Design review of the part shown in the three views and the two pictorial views. Dimensions are in mm from the part's minimum x, y and z. A direction names the side the tool comes from. Round coordinates to 2 decimals unless told otherwise and drop trailing zeros. Order: outer loops, then holes, each group sorted by start corner. A loop starts at its lowest first (then second) coordinate and runs counter-clockwise, first axis right, second up.
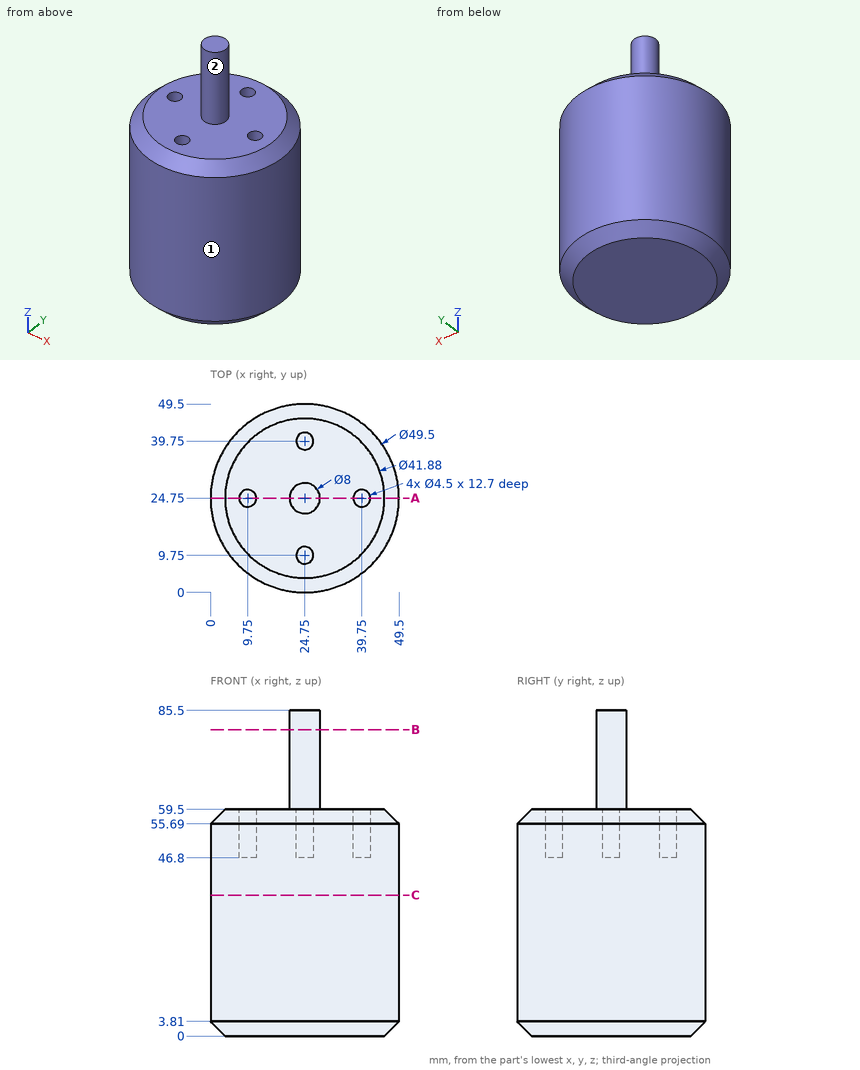
(1) Insertion check: pin 1 (10 mm diameter, centred on y = 38.5, z = 72.5, fed in from -X); pin 2 (1 mm diameter, centred on y = 35, z = 39.5, fed in from +X); pin 3 (3.5 mm diameter, centred on x = 9.75, y = 24.75, fed in from +Z); pin 4 (7 mm diameter, centred on x = 24.75, y = 9.75, fed in from +Z). Each pin has a flat end and moves straight along its axis. Give the tip position at first contact, or say it passes through.
Data:
pin 1: passes through
pin 2: stops at x = 47.5
pin 3: stops at z = 46.8
pin 4: stops at z = 59.5
(2) To check wall thickness, follow probe 1 along Y at (x, z) = (24.75, 54); probe 2 along X at (y, z) = (24, 48.5). State the ranges of each line that lie inside material, in increasing order.
Data:
probe 1: y = 0 to 7.5, 12 to 37.5, 42 to 49.5
probe 2: x = 0.01 to 7.63, 11.87 to 37.63, 41.87 to 49.49
(3) Consider section C-C (z = 37). Write out the cut boundary in (x, y), and give its area (3 significant figures).
Data:
outline: circle Ø49.5 at (24.75, 24.75)
area: 1,920 mm2
(4) Consider section A-A (y = 24.75). Write out the cut boundary in (x, z).
Data:
outline: (0, 3.81) - (3.81, 0) - (45.69, 0) - (49.5, 3.81) - (49.5, 55.69) - (45.69, 59.5) - (42, 59.5) - (42, 46.8) - (37.5, 46.8) - (37.5, 59.5) - (28.75, 59.5) - (28.75, 85.5) - (20.75, 85.5) - (20.75, 59.5) - (12, 59.5) - (12, 46.8) - (7.5, 46.8) - (7.5, 59.5) - (3.81, 59.5) - (0, 55.69) - close
(5) For the marked faces 1 and 2, list the 3-axis set-ups (+Z, -Z, +X, -X, +Y, -Y) from which the entire face can be reached by the end or side of a thin tool; tool diameter is ignored.
Data:
face 1: +Z, -Z
face 2: +Z
(6) Consider section B-B (z = 80.5). Write out the cut boundary in (x, y), and give its area (3 significant figures).
Data:
outline: circle Ø8 at (24.75, 24.75)
area: 50.3 mm2
